Autodesk Inventor part; units mm, degrees
ref_plane "Work Plane1" through (0, 0, 84) normal (0, 0, 1) x (1, 0, 0)
ref_plane "YZ Plane" through (0, 0, 0) normal (1, 0, 0) x (0, 1, 0)
ref_plane "XZ Plane" through (0, 0, 0) normal (0, 1, 0) x (-1, 0, 0)
sketch "Sketch1" plane through (0, 0, 0) normal (0, 0, 1) x (1, 0, 0)
  line L0 (84, 150) -> (84, -150)
  line L1 (-84, 150) -> (-84, -150)
  line L2 (-84, 150) -> (84, 150)
  line L3 (-15.51, 54.8641) -> (15.51, 54.8641)
  line L4 (0, 0) -> (0, 174.1286) construction
  line L5 (15.51, 55.3641) -> (83.5, 108.4837)
  line L6 (15.51, 54.8641) -> (15.51, 55.3641) construction
  line L7 (81.653, 110.8478) -> (13.663, 57.7281)
  line L8 (83.5, 108.4837) -> (81.653, 110.8478)
  line L9 (15.51, 55.3641) -> (13.663, 57.7281)
  line L10 (15.51, 55.3641) -> (0, 55.3641)
  line L11 (13.663, 57.7281) -> (0, 57.7281)
  line L12 (81.653, 110.8478) -> (0, 110.8478)
  line L13 (26.2712, 67.5787) -> (28.1182, 65.2147)
  line L14 (34.1513, 73.7353) -> (35.9983, 71.3713)
  line L15 (53.0636, 88.5112) -> (54.9105, 86.1472)
  line L16 (45.1834, 82.3546) -> (47.0304, 79.9906)
  line L17 (71.9758, 103.2871) -> (73.8228, 100.9231)
  line L18 (64.0957, 97.1305) -> (65.9427, 94.7664)
  dimension "d0" = 0.5
  dimension "d1" = 0.5
  dimension "d2" = 38
  dimension "d3" = 3
  dimension "d4" = 10
  dimension "d5" = 16
  dimension "d8" = 24
extrude "Extrusion1" add sketch "Sketch1" along normal blind 168
sketch "Sketch2" plane through (13.663, 57.7281, 168) normal (-0.6157, 0.788, 0) x (0.788, 0.6157, 0)
  line L0 (-3.8398, 68.49) -> (0, 70.337)
  line L1 (0, 70.337) -> (0, 65.4642)
  line L2 (0, 65.4642) -> (12.5671, 55.5612)
  line L3 (12.5671, 55.5612) -> (14.9359, 58.5673)
  line L4 (14.9359, 58.5673) -> (22.7903, 52.378)
  line L5 (22.7903, 52.378) -> (20.4215, 49.3718)
  line L6 (20.4215, 49.3718) -> (12.5671, 55.5612)
  line L7 (0, 65.4642) -> (-3.8398, 68.49)
  line L8 (20.4215, 49.3718) -> (34.5594, 38.231)
  line L9 (34.5594, 38.231) -> (36.9283, 41.2371)
  line L10 (36.9283, 41.2371) -> (44.7827, 35.0477)
  line L11 (44.7827, 35.0477) -> (42.4138, 32.0416)
  line L12 (42.4138, 32.0416) -> (34.5594, 38.231)
  line L13 (42.4138, 32.0416) -> (56.5518, 20.9008)
  line L14 (56.5518, 20.9008) -> (58.9206, 23.9069)
  line L15 (58.9206, 23.9069) -> (66.775, 17.7175)
  line L16 (66.775, 17.7175) -> (64.4062, 14.7114)
  line L17 (64.4062, 14.7114) -> (56.5518, 20.9008)
  line L18 (64.4062, 14.7114) -> (82.4407, 0.5)
  point P0 (-46.3076, 168)
sketch "Sketch4" plane through (83.5, 108.4837, 0) normal (0.6157, -0.788, 0) x (0.788, 0.6157, 0)
  line L0 (-64.3881, 116.7615) -> (-62.0193, 113.7554)
  line L1 (-62.0193, 113.7554) -> (-69.8737, 107.566)
  line L2 (-69.8737, 107.566) -> (-72.2425, 110.5721)
  line L3 (-72.2425, 110.5721) -> (-64.3881, 116.7615)
  line L4 (-42.3958, 134.0917) -> (-40.0269, 131.0856)
  line L5 (-40.0269, 131.0856) -> (-47.8813, 124.8962)
  line L6 (-47.8813, 124.8962) -> (-50.2502, 127.9023)
  line L7 (-50.2502, 127.9023) -> (-42.3958, 134.0917)
  line L8 (-20.4034, 151.4219) -> (-18.0345, 148.4158)
  line L9 (-18.0345, 148.4158) -> (-25.889, 142.2264)
  line L10 (-25.889, 142.2264) -> (-28.2578, 145.2325)
  line L11 (-28.2578, 145.2325) -> (-20.4034, 151.4219)
  point P0 (-132.5881, 0)
extrude "Extrusion2" cut sketch "Sketch4" against normal blind 10
extrude "Extrusion3" cut sketch "Sketch2" against normal blind 10 contours L14 L15 L16 L17 | L9 L10 L11 L12 | L3 L4 L5 L6
ref_plane "Work Plane1" through (0, 0, 84) normal (0, 0, 1) x (1, 0, 0)
extrude "Extrusion4" add sketch "Sketch1" against normal blind 3 contours L13 L7 L14 L5 | L16 L7 L15 L5 | L18 L7 L17 L5
mirror "Mirror1" about plane through (0, 0, 84) normal (0, 0, 1) of "Extrusion3", "Extrusion2", "Extrusion4"
sketch "Sketch5" plane through (83.5, 108.4837, 0) normal (0.6157, -0.788, 0) x (0.788, 0.6157, 0)
  arc A0 (-87.0927, 88.4093) -> (-87.0927, 79.5907) centre (-115.3496, 84) ccw
  ellipse E0 centre (-105.963, 84) end of major axis (-125.6455, 84) minor radius 15.51 (-87.0927, 88.4093) -> (-92.8236, 95.5479) ccw construction
  arc A1 (-92.8236, 95.5479) -> (-92.8236, 72.4521) centre (-115.3496, 84) ccw construction
  ellipse E1 centre (-105.963, 84) end of major axis (-125.6455, 84) minor radius 15.51 (-92.8236, 72.4521) -> (-87.0927, 79.5907) ccw construction
  ellipse E2 centre (-108.0655, 93.2437) end of major axis (-130.5282, 110.9446) minor radius 17.7588 (-109.3091, 73.4457) -> (-87.7759, 73.4457) ccw
  line L0 (-84.8251, 67.3112) -> (-87.7759, 73.4457)
  ellipse E3 centre (-108.0655, 74.7563) end of major axis (-130.5282, 57.0554) minor radius 17.7588 (-87.7759, 94.5543) -> (-109.3091, 94.5543) ccw
  line L1 (-84.8251, 100.6888) -> (-87.7759, 94.5543)
  line L2 (-86.2805, 0) -> (-86.2805, 168)
  line L3 (-86.2805, 73.4457) -> (-88.7695, 73.4457)
  line L4 (-86.2805, 94.5543) -> (-88.7695, 94.5543)
  circle A2 centre (-115.3496, 84) radius 28.5989
  point P0 (-132.5881, 0)
  point P1 (-87.0927, 79.5907)
  point P2 (-87.0927, 88.4093)
extrude "Extrusion5" add sketch "Sketch5" against normal up to surface (3 mm away) contours A0 L4 L2 L3 A2
chamfer "Chamfer1" distance 30 distance2 8 1 edges at (14.5865, 56.5461, 0) measured on face at (14.2787, 56.9401, 48.9638)
chamfer "Chamfer2" distance 8 distance2 30 1 edges at (14.5865, 56.5461, 168) measured on face at (18.4814, 60.2237, 168)
properties part number "Tolva_Largo"
Could you check a few things on this model? Use its own coordinates, in mm. A direction names the side the tool comes from. Round coordinates to 2 decimals unless told otherwise and drop trailing zeros. Order: outer loops, then holes, each group sorted by start corner. A loop starts at its lowest first (then second) coordinate and runs counter-clockwise, first axis right, second up. Notation, with made-up numbers: M 57,68 L 69,68 A16 ccw 69,89 Z; hole C 30.5,-10.75 d5. An arc over 180 degrees is marked long. One line per item, written item: value.
(1) I need wall thicknesses on line 1 along Y through (x, z) = (69, 105); line 2 along X through (y, z) = (79, 62.5); line 3 along X through (y, z) = (65.5, 80.5). Which ranges of each line are inside material? Lowest first, please. Write a range as from..to.
Ans:
line 1: y = 97.16..100.96
line 2: x = 40.89..45.76
line 3: x = 23.61..28.48
(2) If we mould it in two halves opening along Y, with no side actions, what happens to faces 1 (the flat face through (50, 84, -3)), 2 (the flat face through (43.91, 79.43, 41.58)), 3 (the flat face through (17.77, 59.06, 14.79)), 4 (the flat face through (43.94, 79.45, 126.38))? For each: released by +Y, released by -Y, zero draft, split by the parting line, or undercut.
Ans:
face 1: zero draft
face 2: undercut
face 3: released by -Y
face 4: undercut
(3) Imagine slicing it at A-A (z = 121.5). Write out the boundary of the cut face in (x, y), and give its area (3 significant figures).
Ans:
outline: M 13.66,57.73 L 15.51,55.36 L 83.5,108.48 L 81.65,110.85 Z
area: 259 mm^2
(4) I'm going to push flat-ended pins straight in: P1, Ø10, axis at x = 74, y = 102, coming from the +Z side; P2, Ø1.1, axis at x = 13, y = 56, coming from the +Z side; P3, Ø4, axis at y = 62.5, z = 149, coming from the +X side; P4, Ø12, axis at y = 101.5, z = 118, coming from the +X side. Where does each tip first touch, or does it pass through?
Ans:
P1: stops at z = 171
P2: stops at z = 94.55
P3: stops at x = 27.2
P4: stops at x = 82.24
(5) Which directions (+Z, -Z, +X, -X, +Y, -Y) give clear straight access to the entire face, cutting with the end or side of a thin tool? Please do faces 5 (the flat face through (14, 56, 94.554)), 6 (the flat face through (69, 99, -3)), 7 (the flat face through (48.916, 83.394, 33.524)).
Ans:
face 5: +Z, -X, -Y
face 6: -Z, +X, -X, +Y, -Y
face 7: none
(6) Imagine slicing it at B-B (x = 56.5). Write out the boundary of the cut face in (y, z), and give its area (3 significant figures).
Ans:
outline: M 87.39,0 L 91.2,0 L 91.2,168 L 87.39,168 Z
area: 640 mm^2
